Could you check a few things on this model? Use its own coordinates, in mm. A direction names the side the tool comes from. Give positions to 0.01 mm unless a question says otherwise; leave off trailing zeros. Order: outer loops, then holes, each group sorted by start corner. A loop starts at its lowest first (then second) coordinate and runs counter-clockwise, first axis right, second up.
(1) Imagine slicing it at B-B, the plane y = -14. Write out the boundary of the cut face in (x, z) (3 decimals).
(2) Imagine slicing it at C-C, the plane x = -4. Write out the boundary of the cut face in (y, z) (3 decimals).
(3) Imagine slicing it at A-A, the plane z = 26. Write out the boundary of the cut face in (x, y) (3 decimals), then the cut area to 3 significant figures.
(4) On a 3-axis mill with a long thin cutter (end or side, diameter ignored), from which of +Z, -Z, +X, -X, +Y, -Y can I reach the whole of each face in a straight line? I mean faces 4 (the flat face through (11, 0, 18)), 5 (the flat face through (9, -2.54, 18)), 6 (the flat face through (0, 3.175, 16)), 7 (the flat face through (14.605, 0, 6)), 8 (the flat face through (-13.335, -12, 36)). Say none if no direction works.
(5) If I drill on probe 1 along Z at (x, y) = (6.5, -9); probe 2 along Z at (x, y) = (14.5, -5.5); probe 3 along Z at (x, y) = (7, 10.5), over which ranges is the centre line in solid material (lowest first)?
(6) Imagine slicing it at D-D, the plane x = 11.5. Write out the boundary of the cut face in (y, z) (3 decimals).
(7) Will these pins go through, and if not, where does the flat tip stop? pin 1 (10 mm diameter, centred on x = 2, y = -10.5, fed in from -Z); pin 2 (1.3 mm diameter, centred on x = 14.5, y = -5.5, fed in from +Z); pin 3 (3 mm diameter, centred on x = 6, y = -1.5, fed in from +Z); pin 4 (1.3 mm diameter, centred on x = 14, z = 25.5, fed in from +Y).
(8) If we mould it in two halves opening along Z, with no side actions, what happens to faces 1 (the flat face through (0, 0, 0)), 2 (the flat face through (4.4, -17.78, 34.5)), 3 (the flat face through (15, -15.24, 28))? For each: released by +Z, released by -Z, zero draft, split by the parting line, or undercut.
from build123d import *

# Parameters (mm, degrees)
F0_W      = 29.21
F0_H      = 25.4
F1_DEPTH  = 12.7
F2_W      = 6.35
F2_H      = 6.35
F3_DEPTH  = 7.62
F4_W      = 25.4
F4_H      = 29.21
F5_DEPTH  = 6.35
F6_W      = 25.4
F6_H      = 3.81
F7_DEPTH  = 25.4
F8_W      = 2.54
F8_H      = 2.54
F9_DEPTH  = 12.7
F10_W     = 2.54
F10_H     = 17.78
F11_DEPTH = 2.54
F12_W     = 2.54
F12_H     = 2.54
F13_DEPTH = 12.7
F14_W     = 29.21
F14_H     = 12.7
F15_DEPTH = 2.54


with BuildPart() as f1:
    # F0 (on Top) → F1 (new body)
    with BuildSketch(Plane.XY):
        Rectangle(F0_W, F0_H)
    extrude(amount=F1_DEPTH)

    # F2 (on face) → F3 (join)
    with BuildSketch(Plane.XY.offset(12.7)):
        Rectangle(F2_W, F2_H)
    extrude(amount=F3_DEPTH)

    # F4 (on face) → F5 (join)
    with BuildSketch(Plane.XY.offset(20.32)):
        Rectangle(F4_W, F4_H)
    extrude(amount=F5_DEPTH)

    # F6 (on face) → F7 (join)
    with BuildSketch(Plane.XY.offset(26.67)):
        with Locations((0, 12.7)):
            Rectangle(F6_W, F6_H)
    extrude(amount=F7_DEPTH)

    # F8 (on face) → F9 (join)
    with BuildSketch(Plane.YZ.offset(3.175)):
        with Locations((-1.27, 17.78)):
            Rectangle(F8_W, F8_H)
    extrude(amount=F9_DEPTH)

    # F10 (on face) → F11 (join)
    with BuildSketch(Plane.XY.offset(19.05)):
        with Locations((14.605, -8.89)):
            Rectangle(F10_W, F10_H)
    extrude(amount=F11_DEPTH)

    # F12 (on face) → F13 (join)
    with BuildSketch(Plane.XY.offset(21.59)):
        with Locations((14.605, -16.51)):
            Rectangle(F12_W, F12_H)
    extrude(amount=F13_DEPTH)

    # F14 (on face) → F15 (join)
    with BuildSketch(Plane.XY.offset(34.29)):
        with Locations((1.27, -11.43)):
            Rectangle(F14_W, F14_H)
    extrude(amount=F15_DEPTH)


solid = f1.part
Answer block:
1. outline: (-13.335, 34.29) - (15.875, 34.29) - (15.875, 36.83) - (-13.335, 36.83) - close; (-12.7, 20.32) - (12.7, 20.32) - (12.7, 26.67) - (-12.7, 26.67) - close; (13.335, 19.05) - (15.875, 19.05) - (15.875, 21.59) - (13.335, 21.59) - close
2. outline: (-17.78, 34.29) - (-5.08, 34.29) - (-5.08, 36.83) - (-17.78, 36.83) - close; (-14.605, 20.32) - (14.605, 20.32) - (14.605, 52.07) - (10.795, 52.07) - (10.795, 26.67) - (-14.605, 26.67) - close; (-12.7, 0) - (12.7, 0) - (12.7, 12.7) - (-12.7, 12.7) - close
3. outline: (-12.7, -14.605) - (12.7, -14.605) - (12.7, 14.605) - (-12.7, 14.605) - close; (13.335, -17.78) - (15.875, -17.78) - (15.875, -15.24) - (13.335, -15.24) - close
3. area: 748 mm2
4. face 4: +X, +Y
4. face 5: +X, -Y
4. face 6: +X, -X, +Y
4. face 7: -Z, +X, +Y, -Y
4. face 8: +Z, -X, +Y, -Y
5. probe 1: z = 0 to 12.7, 20.32 to 26.67, 34.29 to 36.83
5. probe 2: z = 0 to 12.7, 19.05 to 21.59, 34.29 to 36.83
5. probe 3: z = 0 to 12.7, 20.32 to 26.67
6. outline: (-17.78, 34.29) - (-5.08, 34.29) - (-5.08, 36.83) - (-17.78, 36.83) - close; (-14.605, 20.32) - (14.605, 20.32) - (14.605, 52.07) - (10.795, 52.07) - (10.795, 26.67) - (-14.605, 26.67) - close; (-12.7, 0) - (12.7, 0) - (12.7, 12.7) - (-12.7, 12.7) - close; (-2.54, 16.51) - (0, 16.51) - (0, 19.05) - (-2.54, 19.05) - close
7. pin 1: stops at z = 0
7. pin 2: stops at z = 36.83
7. pin 3: stops at z = 26.67
7. pin 4: stops at y = -15.24
8. face 1: released by -Z
8. face 2: zero draft
8. face 3: undercut
